from build123d import *

# Parameters (mm, degrees)
CROQUIS3_W              = 76.851762212
CROQUIS3_H              = 62.828734274
SALIENTE_EXTRUIR1_DEPTH = 30
CROQUIS4_W              = 69
CROQUIS4_H              = 55
CORTAR_EXTRUIR1_DEPTH   = 26
REDONDEO5_R             = 2
REDONDEO6_R             = 2
REDONDEO7_R             = 2
CROQUIS5_W              = 3
CROQUIS5_H              = 55
CORTAR_EXTRUIR2_DEPTH   = 70
CROQUIS6_W              = 1.6
CROQUIS6_H              = 57.8
CORTAR_EXTRUIR3_DEPTH   = 73


with BuildPart() as part:
    # Croquis3 → Saliente-Extruir1 (new body)
    with BuildSketch(Plane.XY):
        with Locations((38.425881106, 31.414367137)):
            Rectangle(CROQUIS3_W, CROQUIS3_H)
    extrude(amount=SALIENTE_EXTRUIR1_DEPTH)

    # Croquis4 → Cortar-Extruir1 (cut)
    with BuildSketch(Plane.XY):
        with Locations((38.5, 31.5)):
            Rectangle(CROQUIS4_W, CROQUIS4_H)
    extrude(amount=CORTAR_EXTRUIR1_DEPTH, mode=Mode.SUBTRACT)

    # Redondeo5
    redondeo5_edges = [part.edges().sort_by_distance(p)[0] for p in [
        (0, 0, 15),
        (0, 62.828734274, 15),
        (76.851762212, 62.828734274, 15),
        (76.851762212, 0, 15),
    ]]
    fillet(redondeo5_edges, radius=REDONDEO5_R)

    # Redondeo6
    redondeo6_edges = [part.edges().sort_by_distance(p)[0] for p in [
        (0, 31.414367137, 0),
        (38.425881106, 0, 0),
        (38.425881106, 62.828734274, 0),
        (76.851762212, 31.414367137, 0),
        (76.265975775, 62.242947836, 0),
        (76.265975775, 0.585786438, 0),
        (0.585786438, 0.585786438, 0),
        (0.585786438, 62.242947836, 0),
    ]]
    fillet(redondeo6_edges, radius=REDONDEO6_R)

    # Redondeo7
    redondeo7_edges = [part.edges().sort_by_distance(p)[0] for p in [
        (0, 31.414367137, 30),
        (38.425881106, 62.828734274, 30),
        (38.425881106, 0, 30),
        (76.851762212, 31.414367137, 30),
        (76.265975775, 62.242947836, 30),
        (76.265975775, 0.585786438, 30),
        (0.585786438, 0.585786438, 30),
        (0.585786438, 62.242947836, 30),
    ]]
    fillet(redondeo7_edges, radius=REDONDEO7_R)

    # Croquis5 → Cortar-Extruir2 (cut)
    with BuildSketch(Plane(origin=(0, 0, 0), x_dir=(0, 0, -1), z_dir=(1, 0, 0))):
        with Locations((-1.5, 31.5)):
            Rectangle(CROQUIS5_W, CROQUIS5_H)
    extrude(amount=CORTAR_EXTRUIR2_DEPTH, mode=Mode.SUBTRACT)

    # Croquis6 → Cortar-Extruir3 (cut)
    with BuildSketch(Plane(origin=(0, 0, 0), x_dir=(0, 0, -1), z_dir=(1, 0, 0))):
        with Locations((-2.2, 31.5)):
            Rectangle(CROQUIS6_W, CROQUIS6_H)
    extrude(amount=CORTAR_EXTRUIR3_DEPTH, mode=Mode.SUBTRACT)


solid = part.part
Input: part model. Units: mm. Frame: model coordinates. A direction names the side the tool comes from. Round coordinates to 2 decimals unless told otherwise and drop trailing zeros. Loops run counter-clockwise (first coordinate to the right, second up) from the corner with the lowest first, then second, coordinate; pieces in that order, holes last. Notation, with made-up numbers: (2.5, 61) -> (43.5, 61) arc R18 cw to (43.5, 87) -> close; hole circle Ø9 at (-30, 50). An arc over 180 degrees is marked (long way). Answer as a JSON object with one key per item and string values. Group by question number.
1) Reachability of faces 1 (the flat face through (38, 0, 15)), 2 (the flat face through (38, 59, 15)) from +Z, -Z, +X, -X, +Y, -Y: full face, straight path, thin tool, end or side. Return the list, or none.
2) Pin query (flat end, axial travel): pin 1 (0.7 mm diameter, centred on x = 31, z = 0.5, fed in from +Y); pin 2 (16.5 mm diameter, centred on x = 41.5, y = 44.5, fed in from -Z); pin 3 (1.5 mm diameter, centred on x = 45, z = 0.5, fed in from -Y). Return the tip coordinate at first contact, or that it passes through.
3) Draft query along Y for faces 3 (the flat face through (38, 32, 26)), 4 (the flat face through (0, 31, 15)), 5 (the cylindrical face through (0.57, 0.6, 15.18)). Return one class per face: +Y half, -Y half, draft (parallel to the pull), parting line (faces both ways), or undercut.
4) Ray query, L1, parallel to Y at x = 33, z = 4.5; L2, parallel to X at y = 8.5, z = 21.5; L3, parallel to Y at x = 55.5, z = 28.25. Return the intervals inside material, ascending.
5) Section query C-C on z = 15.5. Output: boundary loops of the cut face in (x, y), plus the area to 3 significant figures.
6) Section query A-A on x = 40.5. Output: boundary loops of the cut face in (y, z), plus the area to 3 significant figures.
7) Section query B-B on y = 19.5. Output: boundary loops of the cut face in (x, z), plus the area to 3 significant figures.
Reply:
{
 "1": {"face 1": "+Z, -Z, +X, -X, -Y", "face 2": "-Z"},
 "2": {"pin 1": "stops at y = 62.47", "pin 2": "stops at z = 26", "pin 3": "stops at y = 0.15"},
 "3": {"face 3": "undercut", "face 4": "draft", "face 5": "-Y half"},
 "4": {"L1": "y = 0 to 4, 59 to 62.83", "L2": "x = 0 to 4, 73 to 76.85", "L3": "y = 0.02 to 62.81"},
 "5": {"outline": "(0, 2) arc R2 ccw to (2, 0) -> (74.85, 0) arc R2 ccw to (76.85, 2) -> (76.85, 60.83) arc R2 ccw to (74.85, 62.83) -> (2, 62.83) arc R2 ccw to (0, 60.83) -> close; hole (4, 4) -> (73, 4) -> (73, 59) -> (4, 59) -> close", "area": "1,030 mm2"},
 "6": {"outline": "(0, 2) arc R2 ccw to (2, 0) -> (4, 0) -> (4, 1.4) -> (2.6, 1.4) -> (2.6, 3) -> (4, 3) -> (4, 26) -> (59, 26) -> (59, 3) -> (60.4, 3) -> (60.4, 1.4) -> (59, 1.4) -> (59, 0) -> (60.83, 0) arc R2 ccw to (62.83, 2) -> (62.83, 28) arc R2 ccw to (60.83, 30) -> (2, 30) arc R2 ccw to (0, 28) -> close", "area": "447 mm2"},
 "7": {"outline": "(0, 3) -> (4, 3) -> (4, 26) -> (73, 26) -> (73, 0) -> (74.85, 0) arc R2 ccw to (76.85, 2) -> (76.85, 28) arc R2 ccw to (74.85, 30) -> (2, 30) arc R2 ccw to (0, 28) -> close", "area": "497 mm2"}
}
